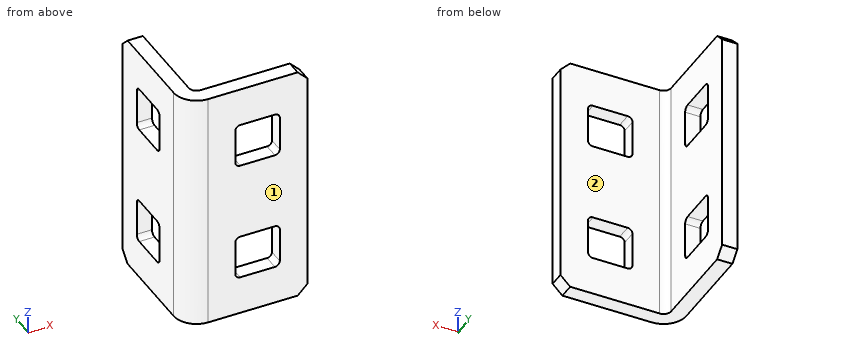
Autodesk Inventor part; units mm, degrees
ref_plane "Diagonal Plane" through (-4.7625, 1.5875, 0) normal (-0.7071068, 0.7071068, 0) x (0, 0, 1)
ref_plane "YZ Plane" through (0, 0, 0) normal (1, 0, 0) x (0, 1, 0)
ref_plane "XZ Plane" through (0, 0, 0) normal (0, 1, 0) x (-1, 0, 0)
sketch "Sketch1" plane through (0, 0, 0) normal (0, 1, 0) x (-1, 0, 0)
  line L0 (-6.35, 0) -> (6.35, 0)
  line L1 (6.35, 0) -> (6.35, -25.4)
  line L2 (6.35, -25.4) -> (-6.35, -25.4)
  line L3 (-6.35, -25.4) -> (-6.35, 0)
  line L4 (6.35, 0) -> (-6.35, -25.4) construction
  point P0 (0, 0)
  point P1 (0, 0)
  dimension "d0" = 12.7
  dimension "d1" = 25.4
extrude "Plate1" add sketch "Sketch1" along normal blind 1.5875
sketch "Sketch2" plane through (-4.7625, 0, 0) normal (-1, 0, 0) x (0, -1, 0)
  line L0 (0, -25.4) -> (0, 0)
  line L1 (0, 0) -> (-12.7, 0)
  line L2 (-12.7, 0) -> (-12.7, -25.4)
  line L3 (-12.7, -25.4) -> (0, -25.4)
edge flange "Flanges" height 12.7 angle 90 thickness 1.5875 bend radius 0.7937 thickness toward (-1, 0, 0) relief tear relief width 1.5875 relief depth 0.7937 edges at (-6.35, 1.5875, -12.7) wall of the first edge with corners at (-4.7625, 0, -25.4) (-4.7625, 0, 0) (-4.7625, 12.7, 0) (-4.7625, 12.7, -25.4)
bend "Bend1"
corner "Corner1"
sketch "Sketch8" plane through (0, 0, 0) normal (0, -1, 0) x (1, 0, 0)
  line L0 (6.35, 0) -> (-3.9687, 0) construction
  line L1 (2.9718, -4.0386) -> (-0.635, -4.0386)
  line L2 (-1.143, -4.5466) -> (-1.143, -8.1534)
  line L3 (-0.635, -8.6614) -> (2.9718, -8.6614)
  line L4 (3.4798, -8.1534) -> (3.4798, -4.5466)
  arc A0 (3.4798, -4.5466) -> (2.9718, -4.0386) centre (2.9718, -4.5466) ccw
  arc A1 (2.9718, -8.6614) -> (3.4798, -8.1534) centre (2.9718, -8.1534) ccw
  arc A2 (-1.143, -8.1534) -> (-0.635, -8.6614) centre (-0.635, -8.1534) ccw
  arc A3 (-0.635, -4.0386) -> (-1.143, -4.5466) centre (-0.635, -4.5466) ccw
  line L5 (2.9718, -4.5466) -> (-0.635, -8.1534) construction
  line L6 (6.35, -25.4) -> (6.35, 0) construction
  point P0 (0, 0)
  point P1 (-1.143, -8.6614)
  point P2 (3.4798, -8.6614)
  point P3 (12.7, 0)
  point P4 (1.1684, -6.35)
  dimension "d49" = 4.6228
  dimension "d50" = 0.508
  dimension "d52" = 6.35
  dimension "d123" = 5.1816
extrude "Body Stamp" cut sketch "Sketch8" against normal blind 1.5875
sketch "Sketch9" plane through (0, 0, 0) normal (0, -1, 0) x (1, 0, 0)
  arc A0 (3.4798, -4.5466) -> (2.9718, -4.0386) centre (2.9718, -4.5466) ccw construction
  arc A1 (-1.143, -8.1534) -> (-0.635, -8.6614) centre (-0.635, -8.1534) ccw construction
  line L0 (2.9718, -4.5466) -> (-0.635, -8.1534) construction
  circle A2 centre (1.1684, -6.35) radius 2.1844
  point P0 (0, 0)
  dimension "d55" = 4.3688
surface extrude "Body Circle" sketch "Sketch9" against normal up to surface (1.5875 mm away) shown yes curves A2
sketch "Body Pattern Sketch" plane through (0, 0, 0) normal (0, -1, 0) x (1, 0, 0)
  line L0 (1.1684, -6.35) -> (1.1684, 0) construction
  circle A0 centre (1.1684, -6.35) radius 2.1844 construction
  point P0 (1.1684, -19.05)
  dimension "d133" = 12.7
pattern_sketch "Body Pattern" of "Body Stamp", "Body Circle" from (1.1684, 0, -6.35) copies at (1.1684, 0, -19.05)
sketch "Arc Length" plane through (19.05, 2.3812, 0) normal (0, 0, 1) x (1, 0, 0)
  line L0 (-25.4, 0) -> (-23.8125, 0)
  arc A0 (-25.4, 0) -> (-23.0187, -2.3813) centre (-23.0187, 0) ccw
  line L1 (-23.0187, -0.7938) -> (-23.0187, -2.3813)
  arc A1 (-23.8125, 0) -> (-23.0187, -0.7938) centre (-23.0187, 0) ccw
  point P0 (-19.05, -2.3812)
  dimension "d126" = 1.2468
  dimension "d127" = 3.7405
feature "Notch" [suppressed]
pattern_linear "Notch Pattern" [suppressed]
ref_plane "Diagonal Plane" through (-4.7625, 1.5875, 0) normal (-0.7071068, 0.7071068, 0) x (0, 0, 1)
mirror "Everything Mirrored" about plane through (-4.7625, 1.5875, 0) normal (-0.7071068, 0.7071068, 0) of "Body Stamp", "Body Circle", "Body Pattern"
chamfer "End Chamfer" distance 1.016 angle 45 4 edges at (-5.5562, 12.7, -25.4) (-5.5562, 12.7, 0) (6.35, 0.7937, 0) (6.35, 0.7937, -25.4)
sketch "Sketch13" plane through (-6.35, 0, 419.1) normal (1, 0, 0) x (0, 0, -1)
  line L0 (480.568, 12.7) -> (482.6, 10.668)
  line L1 (482.6, 10.668) -> (484.632, 12.7)
  line L2 (480.568, 12.7) -> (484.632, 12.7)
  line L3 (482.6, 3.3973) -> (480.3372, 1.1344)
  line L4 (480.3372, 1.1344) -> (482.6, -1.1284)
  line L5 (482.6, -1.1284) -> (484.8628, 1.1344)
  line L6 (484.8628, 1.1344) -> (482.6, 3.3973)
  line L7 (482.6, 3.3973) -> (482.6, -1.1284) construction
  line L8 (482.6, 10.668) -> (482.6, 3.3973) construction
  line L9 (444.5, 12.7) -> (419.1, 12.7)
  line L10 (444.5, 2.3813) -> (419.1, 2.3813) construction
  line L11 (419.1, 12.7) -> (419.1, 2.3813) construction
  point P0 (444.5, -11.9062)
  point P1 (419.1, 0)
  dimension "d86" = 4.5256
  dimension "d128" = 2.032
  dimension "d129" = 1.016
  dimension "d130" = 63.5
equation "\"d53\" = Thickness"
equation "\"d89\" = Thickness"
equation "\"d1\" = 1.27 * Length"
equation "\"d2\" = Thickness"
equation "\"d3\" = BendReliefWidth"
equation "\"d4\" = BendReliefDepth"
equation "\"d5\" = MinimumRemnant"
equation "\"d6\" = TransitionRadius"
equation "\"d10\" = CornerReliefSize"
equation "\"d11\" = GapSize"
equation "\"d12\" = JacobiRadiusSize"
equation "\"BendRadius\" = Thickness"
equation "\"BendReliefWidth\" = Thickness"
equation "\"BendReliefDepth\" = 0.5 * Thickness"
equation "\"CornerReliefSize\" = 4 * Thickness"
equation "\"MinimumRemnant\" = 2 * Thickness"
equation "\"TransitionRadius\" = BendRadius"
equation "\"JacobiRadiusSize\" = BendRadius"
equation "\"GapSize\" = Thickness"
properties part number "Alu C 1x2x1x35"
Here's how the part is built. I have some questions about the finished solid (model axes, mm). Face numbers are marked on the shaded views. A direction names the side the tool comes from. Coordinates: 2 decimals unless noted, no trailing zeros. Loops run counter-clockwise (first coordinate to the right, second up) from the corner with the lowest first, then second, coordinate; pieces in that order, holes last. Notation, with made-up numbers: (54, -18.75) - (90, -18.75) arc R21 cw to (90, -10.75) - close; hole circle Ø8 at (60, 68.25). An arc over 180 degrees is marked (long way). Answer as CSV lines item,"result".
Q1. For pin 1 (3 mm diameter, centred on x = -1, z = -8, fed in from +Y); pin 2 (0.5 mm diameter, centred on y = 0.5, z = -20, fed in from -X); pin 3 (0.5 mm diameter, centred on x = -5.5, z = -19.5, fed in from -Y), each with a flat end and sliding along its axis, tell me the tip position at first contact or that it passes through.
Response:
pin 1,"y = 1.59"
pin 2,"x = -5.7"
pin 3,"y = 0.37"
Q2. For the marked faces 1 and 2, which set-ups out of +Z, -Z, +X, -X, +Y, -Y let a thin tool reach every point of the face, with its end or its side?
Response:
face 1,"+Z, -Z, +X, -X, -Y"
face 2,"+Z, -Z, +X, +Y"
Q3. If we section it at A-A, the plane y = 8.25: Write out the boundary of the cut face in (x, z).
Response:
outline,"(-6.35, -25.4) - (-4.76, -25.4) - (-4.76, -21.36) - (-6.35, -21.36) - close; (-6.35, -16.74) - (-4.76, -16.74) - (-4.76, -8.66) - (-6.35, -8.66) - close; (-6.35, -4.04) - (-4.76, -4.04) - (-4.76, 0) - (-6.35, 0) - close"
Q4. If I drill on L1, parallel to X at y = 5.5, z = -23.25; L2, parallel to Y at x = -0.75, z = -9.75; L3, parallel to X at y = 1.75, z = -14.75, over which ranges is the centre line in solid material (lowest first)? Write a range as [from, to].
Response:
L1,"[-6.35, -4.76]"
L2,"[0, 1.59]"
L3,"[-6.26, -4.45]"
Q5. If we section it at B-B, the plane z = -18: Write out the boundary of the cut face in (x, y), and give its area (3 significant figures).
Response:
outline,"(-6.35, 2.38) arc R2.38 ccw to (-3.97, 0) - (-1.14, 0) - (-1.14, 1.59) - (-3.97, 1.59) arc R0.79 cw to (-4.76, 2.38) - (-4.76, 5.21) - (-6.35, 5.21) - close; (-6.35, 9.83) - (-4.76, 9.83) - (-4.76, 12.7) - (-6.35, 12.7) - close; (3.48, 0) - (6.35, 0) - (6.35, 1.59) - (3.48, 1.59) - close"
area,"22.0 mm2"
Q6. If we section it at C-C, the plane x = 2.5: Write out the boundary of the cut face in (y, z), and give its area (3 significant figures).
Response:
outline,"(0, -25.4) - (1.59, -25.4) - (1.59, -21.36) - (0, -21.36) - close; (0, -16.74) - (1.59, -16.74) - (1.59, -8.66) - (0, -8.66) - close; (0, -4.04) - (1.59, -4.04) - (1.59, 0) - (0, 0) - close"
area,"25.6 mm2"
Q7. If we section it at D-D, the plane z = -9.75: Write out the boundary of the cut face in (x, y), and give its area (3 significant figures).
Response:
outline,"(-6.35, 2.38) arc R2.38 ccw to (-3.97, 0) - (6.35, 0) - (6.35, 1.59) - (-3.97, 1.59) arc R0.79 cw to (-4.76, 2.38) - (-4.76, 12.7) - (-6.35, 12.7) - close"
area,"36.7 mm2"
